Source: CAD feature listing. Evaluate the final solid. Frame: model axes, mm. Face numbers are marked on the shaded views. A direction names the side the tool comes from. Round coordinates to 2 decimals unless told otherwise and drop trailing zeros. Loops run counter-clockwise (first coordinate to the right, second up) from the corner with the lowest first, then second, coordinate; pieces in that order, holes last. Notation, with made-up numbers: (11.5, -37.75) -> (48.5, -37.75) arc R19 ccw to (48.5, -26.75) -> close; hole circle Ø3 at (11, 32). An arc over 180 degrees is marked (long way). Put each result on its own line as item: value. Start each with the question number.
1. Material intervals for L1, parallel to X at y = -1.05, z = 0; L2, parallel to X at y = -3.55, z = 0; L3, parallel to Y at x = -8.5, z = -1.75, sorted ascending.
2. Draft query along X for the marked faces 1, 2 and 3. Return one class per face: pulls with the +X half, pulls with the -X half, needs draft (parallel to the pull), parting line crosses it, or undercut.
3. Cut plane D-D (y = -8). Return the cut outline in (x, z).
4. Cut plane B-B (z = 0). Return the cut outline in (x, y).
5. Cut plane C-C (x = -5.5). Return the cut outline in (y, z), then the cut area to 3 significant figures.
6. Contact query for flat-ended pins moving along their axis: pin 1 (5.5 mm diameter, centred on x = 19.5, y = -12.5, fed in from -Z); pin 2 (1.5 mm diameter, centred on x = 21, z = -1, fed in from +Y); pin 3 (1 mm diameter, centred on y = -6, z = 0.5, fed in from +X). Output: stop coordinate, or through.
7. Cut plane A-A (y = -12.5). Return the cut outline in (x, z).
8. Set-up query: the marked faces 4 and 5. Return all of +Z, -Z, +X, -X, +Y, -Y with unobstructed straight access to the full face (end or side cutting, diameter ignored); none if empty.
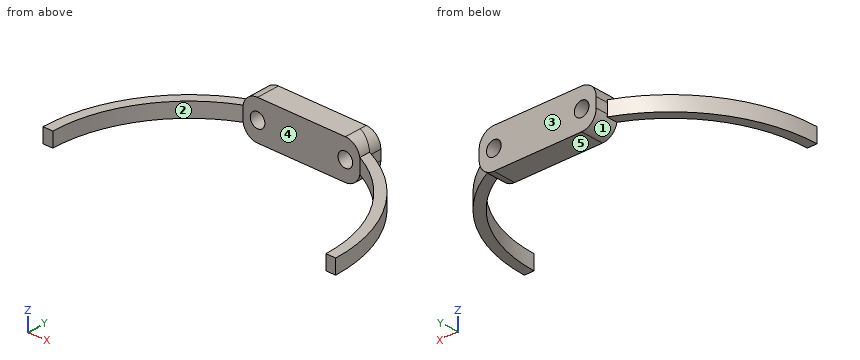
```python
from build123d import *

# Parameters (mm, degrees)
SKETCH_2_W           = 24
SKETCH_2_H           = 8
EXTRUDE_1_DEPTH      = 1
EXTRUDE_3_DEPTH      = 1.5
EXTRUDE_3_DEPTH_BACK = 1.5
EXTRUDE_5_REACH      = 45.174
SKETCH_7_W           = 24
SKETCH_7_H           = 4.701778719
SKETCH_3_R           = 1.5
CUT_EXTRUDE_1_DEPTH  = 43.614551505
FILLET_1_R           = 3


with BuildPart() as part:
    # Sketch 2 → Extrude 1 (new body)
    with BuildSketch(Plane(origin=(0, 0, 0), x_dir=(1, 0, 0), z_dir=(0, 1, 0))):
        Rectangle(SKETCH_2_W, SKETCH_2_H)
    extrude(amount=-EXTRUDE_1_DEPTH)

    # Extrude 5: up to this face of the body (flat: up to its plane)
    extrude_5_end = Plane(part.part.faces().sort_by_distance((0, -0.5, -4))[0])
    # Sketch 7 → Extrude 5 (add, up to the picked face)
    with BuildSketch(Plane.XY.offset(4), mode=Mode.PRIVATE) as extrude_5_sk1:
        with Locations((0, -2.350889359)):
            Rectangle(SKETCH_7_W, SKETCH_7_H)
    extrude_5_tool1 = split(extrude(extrude_5_sk1.sketch, amount=-EXTRUDE_5_REACH, mode=Mode.PRIVATE), bisect_by=extrude_5_end, keep=Keep.BOTH, mode=Mode.PRIVATE)


with BuildPart() as body_2:
    # Sketch 5 → Extrude 3 (new, two sides: drawn at the far end of the back side and taken through both)
    with BuildSketch(Plane.XY.offset(-EXTRUDE_3_DEPTH_BACK)):
        with BuildLine():
            ThreePointArc((30, -30), (21.213203436, -8.786796564), (0, 0))
            Line((0, 0), (0, -2))
            ThreePointArc((0, -2), (19.798989873, -10.201010127), (28, -30))
            Line((28, -30), (30, -30))
        make_face()
        with BuildLine():
            Line((0, -2), (0, 0))
            ThreePointArc((0, 0), (-21.213203436, -8.786796564), (-30, -30))
            Line((-30, -30), (-28, -30))
            ThreePointArc((-28, -30), (-19.798989873, -10.201010127), (0, -2))
        make_face()
    extrude(amount=EXTRUDE_3_DEPTH + EXTRUDE_3_DEPTH_BACK)


with BuildPart() as part_1:
    add(part.part)

    add(body_2.part)  # Extrude 5 merges body 2
    add(extrude_5_tool1.solids().sort_by(Axis((0, -2.350889, 4), (0, 0, -1)))[0])

    # Sketch 3 → Cut-Extrude 1 (cut, through all)
    with BuildSketch(Plane(origin=(0, 0, 0), x_dir=(1, 0, 0), z_dir=(0, 1, 0))):
        with Locations(Location((-9, 0, 0), (0, 0, 270))):
            Circle(SKETCH_3_R)
        with Locations(Location((9, 0, 0), (0, 0, 270))):
            Circle(SKETCH_3_R)
    extrude(amount=-CUT_EXTRUDE_1_DEPTH, mode=Mode.SUBTRACT)

    # Fillet 1
    # the kernel refuses this fillet: 3 mm, written as the material it takes off along each edge
    with BuildSketch(Plane(origin=(-12, -12.201778719, 4), x_dir=(0, 0, -1), z_dir=(0, 1, 0))) as fillet_1_piece_1_section:
        with BuildLine():
            CenterArc((FILLET_1_R, -FILLET_1_R), FILLET_1_R, 90, 90)
            Line((0, -FILLET_1_R), (0, 0))
            Line((0, 0), (FILLET_1_R, 0))
        make_face()
    fillet_1_piece_1 = extrude(amount=19.701778719, mode=Mode.PRIVATE)
    fillet_1_piece_1 = split(fillet_1_piece_1, bisect_by=Plane(origin=(-10.876445005, -4.454369233, 1.5), z_dir=(0, 0, 1)), keep=Keep.TOP, mode=Mode.PRIVATE)
    add(fillet_1_piece_1, mode=Mode.SUBTRACT)
    with BuildSketch(Plane(origin=(-12, -12.201778719, 4), x_dir=(0, 0, -1), z_dir=(0, 1, 0))) as fillet_1_piece_2_section:
        with BuildLine():
            CenterArc((FILLET_1_R, -FILLET_1_R), FILLET_1_R, 90, 90)
            Line((0, -FILLET_1_R), (0, 0))
            Line((0, 0), (FILLET_1_R, 0))
        make_face()
    fillet_1_piece_2 = extrude(amount=19.701778719, mode=Mode.PRIVATE)
    fillet_1_piece_2 = fillet_1_piece_2 - Plane(origin=(0, -30, 1.375084053), x_dir=(1, 0, 0), z_dir=(0, 0, -1)) * Cylinder(30, 52, mode=Mode.PRIVATE)
    add(fillet_1_piece_2, mode=Mode.SUBTRACT)
    with BuildSketch(Plane(origin=(-12, -12.201778719, -4), x_dir=(1, 0, 0), z_dir=(0, 1, 0))) as fillet_1_piece_3_section:
        with BuildLine():
            CenterArc((FILLET_1_R, -FILLET_1_R), FILLET_1_R, 90, 90)
            Line((0, -FILLET_1_R), (0, 0))
            Line((0, 0), (FILLET_1_R, 0))
        make_face()
    fillet_1_piece_3 = extrude(amount=19.701778719, mode=Mode.PRIVATE)
    fillet_1_piece_3 = split(fillet_1_piece_3, bisect_by=Plane(origin=(-10.876427582, -4.45436464, -1.5), z_dir=(0, 0, -1)), keep=Keep.TOP, mode=Mode.PRIVATE)
    add(fillet_1_piece_3, mode=Mode.SUBTRACT)
    with BuildSketch(Plane(origin=(-12, -12.201778719, -4), x_dir=(1, 0, 0), z_dir=(0, 1, 0))) as fillet_1_piece_4_section:
        with BuildLine():
            CenterArc((FILLET_1_R, -FILLET_1_R), FILLET_1_R, 90, 90)
            Line((0, -FILLET_1_R), (0, 0))
            Line((0, 0), (FILLET_1_R, 0))
        make_face()
    fillet_1_piece_4 = extrude(amount=19.701778719, mode=Mode.PRIVATE)
    fillet_1_piece_4 = fillet_1_piece_4 - Plane(origin=(0, -30, -1.375084091), x_dir=(1, 0, 0), z_dir=(0, 0, -1)) * Cylinder(30, 52, mode=Mode.PRIVATE)
    add(fillet_1_piece_4, mode=Mode.SUBTRACT)
    with BuildSketch(Plane(origin=(12, 7.5, 4), x_dir=(0, 0, -1), z_dir=(0, -1, 0))) as fillet_1_piece_5_section:
        with BuildLine():
            CenterArc((FILLET_1_R, -FILLET_1_R), FILLET_1_R, 90, 90)
            Line((0, -FILLET_1_R), (0, 0))
            Line((0, 0), (FILLET_1_R, 0))
        make_face()
    fillet_1_piece_5 = extrude(amount=19.701778719, mode=Mode.PRIVATE)
    fillet_1_piece_5 = fillet_1_piece_5 - Plane(origin=(0, -30, 1.375084091), x_dir=(1, 0, 0), z_dir=(0, 0, -1)) * Cylinder(30, 52, mode=Mode.PRIVATE)
    add(fillet_1_piece_5, mode=Mode.SUBTRACT)
    with BuildSketch(Plane(origin=(12, 7.5, 4), x_dir=(0, 0, -1), z_dir=(0, -1, 0))) as fillet_1_piece_6_section:
        with BuildLine():
            CenterArc((FILLET_1_R, -FILLET_1_R), FILLET_1_R, 90, 90)
            Line((0, -FILLET_1_R), (0, 0))
            Line((0, 0), (FILLET_1_R, 0))
        make_face()
    fillet_1_piece_6 = extrude(amount=19.701778719, mode=Mode.PRIVATE)
    fillet_1_piece_6 = split(fillet_1_piece_6, bisect_by=Plane(origin=(11.332354587, -3.316124118, 1.5), z_dir=(0, 0, 1)), keep=Keep.TOP, mode=Mode.PRIVATE)
    add(fillet_1_piece_6, mode=Mode.SUBTRACT)
    with BuildSketch(Plane(origin=(12, 7.5, -4), x_dir=(-1, 0, 0), z_dir=(0, -1, 0))) as fillet_1_piece_7_section:
        with BuildLine():
            CenterArc((FILLET_1_R, -FILLET_1_R), FILLET_1_R, 90, 90)
            Line((0, -FILLET_1_R), (0, 0))
            Line((0, 0), (FILLET_1_R, 0))
        make_face()
    fillet_1_piece_7 = extrude(amount=19.701778719, mode=Mode.PRIVATE)
    fillet_1_piece_7 = split(fillet_1_piece_7, bisect_by=Plane(origin=(11.383708583, -1.124807359, -1.5), z_dir=(0, 0, -1)), keep=Keep.TOP, mode=Mode.PRIVATE)
    add(fillet_1_piece_7, mode=Mode.SUBTRACT)
    with BuildSketch(Plane(origin=(12, 7.5, -4), x_dir=(-1, 0, 0), z_dir=(0, -1, 0))) as fillet_1_piece_8_section:
        with BuildLine():
            CenterArc((FILLET_1_R, -FILLET_1_R), FILLET_1_R, 90, 90)
            Line((0, -FILLET_1_R), (0, 0))
            Line((0, 0), (FILLET_1_R, 0))
        make_face()
    fillet_1_piece_8 = extrude(amount=19.701778719, mode=Mode.PRIVATE)
    fillet_1_piece_8 = fillet_1_piece_8 - Plane(origin=(0, -30, -1.375084091), x_dir=(1, 0, 0), z_dir=(0, 0, -1)) * Cylinder(30, 52, mode=Mode.PRIVATE)
    add(fillet_1_piece_8, mode=Mode.SUBTRACT)


solid = part_1.part
```
Solution:
1. L1: x = -12 to -10.5, -7.5 to 7.5, 10.5 to 12
1. L2: x = -14.16 to -10.5, -7.5 to 7.5, 10.5 to 14.16
1. L3: y = -4.7 to 0
2. face 1: pulls with the -X half
2. face 2: undercut
2. face 3: needs draft
3. outline: (-20.4, -1.5) -> (-17.32, -1.5) -> (-17.32, 1.5) -> (-20.4, 1.5) -> close; (17.32, -1.5) -> (20.4, -1.5) -> (20.4, 1.5) -> (17.32, 1.5) -> close
4. outline: (-30, -30) -> (-28, -30) arc R28 cw to (-12, -4.7) -> (-10.5, -4.7) -> (-10.5, 0) -> (-12, 0) -> (-12, -2.5) arc R30 ccw to start; (-7.5, -4.7) -> (7.5, -4.7) -> (7.5, 0) -> (-7.5, 0) -> close; (10.5, -4.7) -> (12, -4.7) arc R28 cw to (28, -30) -> (30, -30) arc R30 ccw to (12, -2.5) -> (12, 0) -> (10.5, 0) -> close
5. outline: (-4.7, -4) -> (0, -4) -> (0, 4) -> (-4.7, 4) -> close
5. area: 37.6 mm^2
6. pin 1: stops at z = -1.5
6. pin 2: stops at y = -7.87
6. pin 3: stops at x = 18.65
7. outline: (-24.37, -1.5) -> (-21.86, -1.5) -> (-21.86, 1.5) -> (-24.37, 1.5) -> close; (21.86, -1.5) -> (24.37, -1.5) -> (24.37, 1.5) -> (21.86, 1.5) -> close
8. face 4: +Z, -Z, -Y
8. face 5: -Z, +X, -X, +Y, -Y
